CAD build for the part. Positions are in the model's coordinates, mm. Face numbers are marked on the shaded views. A direction names the side the tool comes from. Give positions to 0.01 mm unless a question says otherwise; leave off trailing zeros. Write each loop counter-clockwise with the first axis right and the second up, starting at its lowest first coordinate (ties: lowest second). Pieces come first, ordered by that corner, then holes. Notation, with made-up numbers: (-33.75, 66) - (-4.75, 66) arc R30 cw to (-4.75, 95) - close; hole circle Ø3 at (44.25, 35). An arc over 180 degrees is marked (long way). Answer as a JSON object with one key per item and string values.
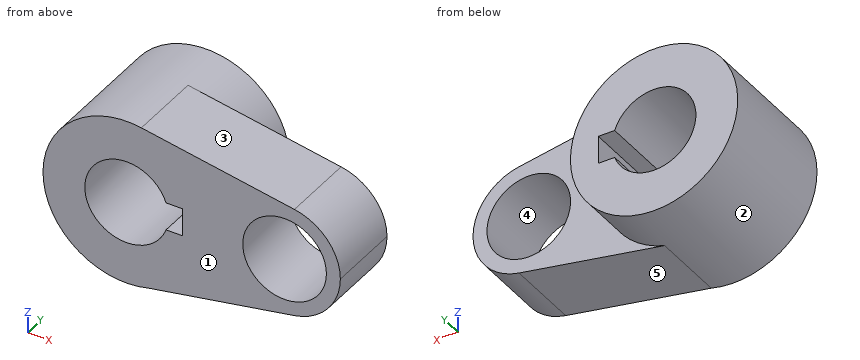
from build123d import *

# Parameters (mm, degrees)
F0_R     = 14.2875
F1_DEPTH = 25.4
F2_DEPTH = 43.18


with BuildPart() as f1:
    # F0 (on Front) → F1 (new body)
    with BuildSketch(Plane.XZ):
        with BuildLine():
            ThreePointArc((7.5618183068, -27.5562974453), (22.7223412429, -17.3270260992), (28.575, 0))
            ThreePointArc((28.575, 0), (21.9160245563, 18.3362616868), (5.0426470588, 28.1265414802))
            ThreePointArc((5.0426470588, 28.1265414802), (-28.5458013461, -1.2914528675), (7.5618183068, -27.5562974453))
        make_face()
        with BuildLine():
            ThreePointArc((-13.4703841816, 4.7625), (0, 14.2875), (13.4703841816, 4.7625))
            Line((13.4703841816, 4.7625), (19.05, 4.7625))
            Line((19.05, 4.7625), (19.05, -4.7625))
            Line((19.05, -4.7625), (13.4703841816, -4.7625))
            ThreePointArc((13.4703841816, -4.7625), (0, -14.2875), (-13.4703841816, -4.7625))
            Line((-13.4703841816, -4.7625), (-19.05, -4.7625))
            Line((-19.05, -4.7625), (-19.05, 4.7625))
            Line((-19.05, 4.7625), (-13.4703841816, 4.7625))
        make_face(mode=Mode.SUBTRACT)
        with BuildLine():
            ThreePointArc((5.0426470588, 28.1265414802), (21.9160245563, 18.3362616868), (28.575, 0))
            ThreePointArc((28.575, 0), (22.7223412429, -17.3270260992), (7.5618183068, -27.5562974453))
            Line((7.5618183068, -27.5562974453), (57.2934332861, -18.7587446415))
            ThreePointArc((57.2934332861, -18.7587446415), (34.9250127111, 0.0220066118), (57.3367647059, 18.7510276535))
            Line((57.3367647059, 18.7510276535), (5.0426470588, 28.1265414802))
        make_face()
        with BuildLine():
            ThreePointArc((73.025, 0), (68.5856830375, 12.2241744579), (57.3367647059, 18.7510276535))
            ThreePointArc((57.3367647059, 18.7510276535), (34.9250127111, 0.0220066118), (57.2934332861, -18.7587446415))
            ThreePointArc((57.2934332861, -18.7587446415), (68.571551889, -12.2410446021), (73.025, 0))
        make_face()
        with Locations((53.975, 0)):
            Circle(F0_R, mode=Mode.SUBTRACT)
        with BuildLine():
            ThreePointArc((-13.4703841816, -4.7625), (-14.2875, 0), (-13.4703841816, 4.7625))
            Line((-13.4703841816, 4.7625), (-19.05, 4.7625))
            Line((-19.05, 4.7625), (-19.05, -4.7625))
            Line((-19.05, -4.7625), (-13.4703841816, -4.7625))
        make_face()
    extrude(amount=-F1_DEPTH)

    # F0 (on Front) → F2 (join)
    with BuildSketch(Plane.XZ):
        with BuildLine():
            ThreePointArc((7.5618183068, -27.5562974453), (22.7223412429, -17.3270260992), (28.575, 0))
            ThreePointArc((28.575, 0), (21.9160245563, 18.3362616868), (5.0426470588, 28.1265414802))
            ThreePointArc((5.0426470588, 28.1265414802), (-28.5458013461, -1.2914528675), (7.5618183068, -27.5562974453))
        make_face()
        with BuildLine():
            ThreePointArc((-13.4703841816, 4.7625), (0, 14.2875), (13.4703841816, 4.7625))
            Line((13.4703841816, 4.7625), (19.05, 4.7625))
            Line((19.05, 4.7625), (19.05, -4.7625))
            Line((19.05, -4.7625), (13.4703841816, -4.7625))
            ThreePointArc((13.4703841816, -4.7625), (0, -14.2875), (-13.4703841816, -4.7625))
            Line((-13.4703841816, -4.7625), (-19.05, -4.7625))
            Line((-19.05, -4.7625), (-19.05, 4.7625))
            Line((-19.05, 4.7625), (-13.4703841816, 4.7625))
        make_face(mode=Mode.SUBTRACT)
        with BuildLine():
            ThreePointArc((-13.4703841816, -4.7625), (-14.2875, 0), (-13.4703841816, 4.7625))
            Line((-13.4703841816, 4.7625), (-19.05, 4.7625))
            Line((-19.05, 4.7625), (-19.05, -4.7625))
            Line((-19.05, -4.7625), (-13.4703841816, -4.7625))
        make_face()
    extrude(amount=-F2_DEPTH)


solid = f1.part
(1) Pull direction Z, two halves, no side cores. Call the marked faces 3, 4 and 5: pulls with the +Z half, pulls with the -Z half, needs draft (parallel to the pull), parting line crosses it, or undercut.
Answer key:
{"face 3": "pulls with the +Z half", "face 4": "undercut", "face 5": "pulls with the -Z half"}
(2) Saw through at B-B, the plane x = 0. Give the cut face in (y, z) (1 decimal), and give its area (3 significant figures).
Answer key:
{"outline": "(0, -28.6) - (43.2, -28.6) - (43.2, -14.3) - (0, -14.3) - close; (0, 14.3) - (43.2, 14.3) - (43.2, 28.6) - (0, 28.6) - close", "area": "1,230 mm²"}
(3) Flat gauge pins, fed straight in: P1, Ø7.5, axis at y = 20, z = 0, coming from the -X side (3 decimals); P2, Ø4.5, axis at x = 17.5, y = 23.5, coming from the -Z side; P3, Ø4.5, axis at x = 17.5, y = 11.5, coming from the +Z side. Where does each tip first touch, or does it go through?
Answer key:
{"P1": "stops at x = -28.575", "P2": "stops at z = -26.2", "P3": "stops at z = 26.3"}
(4) Probe L1, parallel to X at y = 24, z = -2.5; L2, parallel to Z at x = 0, y = 17 (1 decimal); L3, parallel to X at y = 2.5, z = 11.5. List the from-to ranges inside material, lowest first. Write a range as [from, to].
Answer key:
{"L1": "x = [-28.47, -14.07], [19.05, 39.91], [68.04, 72.86]", "L2": "z = [-28.6, -14.3], [14.3, 28.6]", "L3": "x = [-26.16, -8.48], [8.48, 45.5], [62.45, 69.16]"}
(5) 3-axis set-ups, long thin cutter, end or side, ignore diameter. For the marked faces 1 and 2: which of +Z, -Z, +X, -X, +Y, -Y reach the whole face in a straight line?
Answer key:
{"face 1": "+Z, -Z, +X, -X, -Y", "face 2": "+Y"}
(6) Saw through at D-D, the plane z = -12. Give the cut face in (x, y), and give its area (3 significant figures).
Answer key:
{"outline": "(-25.93, 0) - (-7.75, 0) - (-7.75, 43.18) - (-25.93, 43.18) - close; (7.75, 0) - (46.22, 0) - (46.22, 25.4) - (25.93, 25.4) - (25.93, 43.18) - (7.75, 43.18) - close; (61.73, 0) - (68.77, 0) - (68.77, 25.4) - (61.73, 25.4) - close", "area": "2,260 mm²"}
(7) Saw through at C-C, the plane y = 15.5. State how many separate pieces and enclosed holes the cut face has, and give its area (3 significant figures).
Answer key:
{"separate pieces": "1", "enclosed holes": "2", "area": "3,130 mm²"}
